Read the model definition and answer for the solid it produces. Units are mm, in the model's axes. Coordinates: 2 decimals unless noted, no trailing zeros. Loops run counter-clockwise (first coordinate to the right, second up) from the corner with the lowest first, then second, coordinate; pieces in that order, holes last.
from build123d import *

# Parameters (mm, degrees)
SKETCH1_W           = 90
SKETCH1_H           = 35
BOSS_EXTRUDE1_DEPTH = 5
SKETCH2_R           = 1.435
BOSS_EXTRUDE2_DEPTH = 3.5
BOSS_EXTRUDE3_START = 3.5
SKETCH3_R           = 1.435
BOSS_EXTRUDE3_DEPTH = 3.5


with BuildPart() as part:
    # Sketch1 → Boss-Extrude1 (new body)
    with BuildSketch(Plane.XY):
        Rectangle(SKETCH1_W, SKETCH1_H)
    extrude(amount=BOSS_EXTRUDE1_DEPTH)

    # Sketch2 → Boss-Extrude2 (add)
    with BuildSketch(Plane(origin=(45, 0, 0), x_dir=(0, 0, -1), z_dir=(1, 0, 0))):
        with Locations(Location((-2.5, 9.5, 0), (0, 0, 180))):
            Circle(SKETCH2_R)
        with Locations(Location((-2.5, -9.5, 0), (0, 0, 180))):
            Circle(SKETCH2_R)
    extrude(amount=BOSS_EXTRUDE2_DEPTH)

    # Sketch3 → Boss-Extrude3 (add)
    with BuildSketch(Plane.ZY.offset(45).offset(BOSS_EXTRUDE3_START)):
        with Locations((2.5, 9.5)):
            Circle(SKETCH3_R)
        with Locations((2.5, -9.5)):
            Circle(SKETCH3_R)
    extrude(amount=-BOSS_EXTRUDE3_DEPTH)


solid = part.part
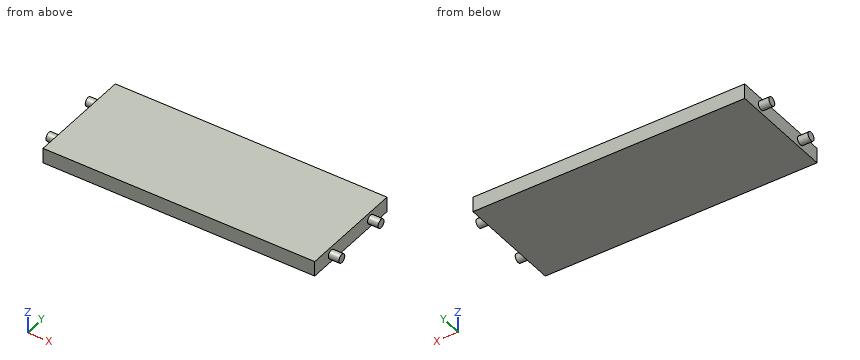
Q1. A cutting plane is placed at B-B (z = 2.5). Give the vertices of the cut face in (x, y) (3 decimals), then the cut area to 3 significant figures.
Findings below:
outline: (-48.5, -10.935) - (-45, -10.935) - (-45, -17.5) - (45, -17.5) - (45, -10.935) - (48.5, -10.935) - (48.5, -8.065) - (45, -8.065) - (45, 8.065) - (48.5, 8.065) - (48.5, 10.935) - (45, 10.935) - (45, 17.5) - (-45, 17.5) - (-45, 10.935) - (-48.5, 10.935) - (-48.5, 8.065) - (-45, 8.065) - (-45, -8.065) - (-48.5, -8.065) - close
area: 3,190 mm2
Q2. A straight line is drawn through the part: probe 1 along X at (y, z) = (14, 2.35). Find the intervals that lie inside material, in ascending order.
Findings below:
probe 1: x = -45 to 45
Q3. Flat-ended cylindrical pins translate along their axes: pin 1 Ø3 at (y, z) = (2.5, 4) entering from -X; pin 2 Ø8 at (x, y) = (36.5, 5.5) entering from -Z. Find the tip coordinate at first contact, or state that the pin passes through.
Findings below:
pin 1: stops at x = -45
pin 2: stops at z = 0
Q4. A cutting plane is placed at C-C (y = 13.5). Give the vertices of the cut face in (x, z).
Findings below:
outline: (-45, 0) - (45, 0) - (45, 5) - (-45, 5) - close
Q5. A cutting plane is placed at A-A (y = 9.5). Give the vertices of the cut face in (x, z) (3 decimals), then the cut area to 3 significant figures.
Findings below:
outline: (-48.5, 1.065) - (-45, 1.065) - (-45, 0) - (45, 0) - (45, 1.065) - (48.5, 1.065) - (48.5, 3.935) - (45, 3.935) - (45, 5) - (-45, 5) - (-45, 3.935) - (-48.5, 3.935) - close
area: 470 mm2
